from build123d import *

# Parameters (mm, degrees)
SKETCH1_R           = 79.5
BOSS_EXTRUDE1_DEPTH = 37
SKETCH2_W           = 80
SKETCH2_H           = 31
BOSS_EXTRUDE2_DEPTH = 212.65
BOSS_EXTRUDE3_DEPTH = 31
CUT_EXTRUDE1_DEPTH  = 10
SKETCH5_R           = 27.5
CUT_EXTRUDE2_DEPTH  = 181


with BuildPart() as part:
    # Sketch1 → Boss-Extrude1 (new body)
    with BuildSketch(Plane.XY):
        with BuildLine():
            ThreePointArc((-21.261874522, 100), (-28.188531545, 98.000973706), (-32.984947104, 92.618680381))
            Line((-32.984947104, 92.618680381), (-71.691097716, 11.860391562))
            ThreePointArc((-71.691097716, 11.860391562), (0, 57), (71.691097716, 11.860391562))
            Line((71.691097716, 11.860391562), (32.984947104, 92.618680381))
            ThreePointArc((32.984947104, 92.618680381), (28.188531545, 98.000973706), (21.261874522, 100))
            Line((21.261874522, 100), (-21.261874522, 100))
        make_face()
        with Locations((0, -22.5)):
            Circle(SKETCH1_R)
    extrude(amount=BOSS_EXTRUDE1_DEPTH)

    # Sketch2 → Boss-Extrude2 (add)
    with BuildSketch(Plane.XY.offset(37)):
        with Locations((0, 62.5)):
            Rectangle(SKETCH2_W, SKETCH2_H)
    extrude(amount=BOSS_EXTRUDE2_DEPTH)

    # Sketch3 → Boss-Extrude3 (add)
    with BuildSketch(Plane(origin=(0, 78, 0), x_dir=(1, 0, 0), z_dir=(0, 1, 0))):
        Polygon((5, -278.784714132), (40, -270.85), (40, -249.65), (-40, -249.65), (-40, -270.85), align=None)
    extrude(amount=-BOSS_EXTRUDE3_DEPTH)

    # Sketch4 → Cut-Extrude1 (cut)
    with BuildSketch(Plane.XY.offset(37)):
        Polygon((55, -22.5), (15, 15), (15, -7.5), (-50, -7.5), (-50, -37.5), (15, -37.5), (15, -60), align=None)
    extrude(amount=-CUT_EXTRUDE1_DEPTH, mode=Mode.SUBTRACT)

    # Sketch5 → Cut-Extrude2 (cut, through all)
    with BuildSketch(Plane(origin=(0, 78, 0), x_dir=(1, 0, 0), z_dir=(0, 1, 0))):
        with Locations((0, -206.1)):
            Circle(SKETCH5_R)
    extrude(amount=-CUT_EXTRUDE2_DEPTH, mode=Mode.SUBTRACT)


solid = part.part
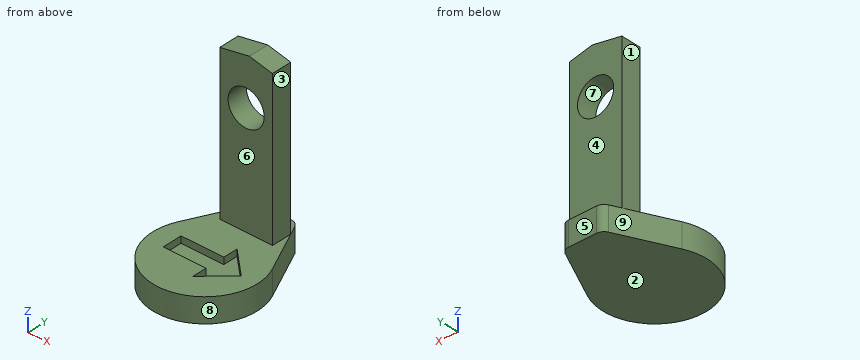
Read the model definition and answer for the solid it produces. Units are mm, in the model's axes. Face numbers are marked on the shaded views. A direction names the side the tool comes from. Round coordinates to 2 decimals unless told otherwise and drop trailing zeros. Order: outer loops, then holes, each group sorted by start corner. A loop starts at its lowest first (then second) coordinate and runs counter-clockwise, first axis right, second up.
1) Straight lines are drawn through the part: L1, parallel to X at y = 57.5, z = 206.1; L2, parallel to Y at x = -12.5, z = 155; L3, parallel to Z at x = 45, y = 19. For each, find the intervals that lie inside material, in ascending order.
2) The mould has two halves that part along X. Classify the marked faces 6, 7, 8 and 9: released by +X, released by -X, zero draft, split by the parting line, or undercut.
3) The part is cut by section C-C on z = 145. Write down the section's boundary in (x, y), plus the area to 3 significant figures.
4) For the marked faces 1, 2, 3, 4 and 5, determine the directions among +Z, -Z, +X, -X, +Y, -Y from which every point of the face is accessible in a straight line to the end or side of a thin tool.
5) Flat-ended cylindrical pins translate along their axes: pin 1 (15.5 mm diameter, centred on y = 55, z = 205, fed in from -X); pin 2 (5 mm diameter, centred on y = -47.5, z = 32.5, fed in from +X); pin 3 (5 mm diameter, centred on y = -1, z = 31, fed in from +X); pin 4 (5 mm diameter, centred on y = -25, z = 29.5, fed in from +X). Find the tip coordinate at first contact, or state that the pin passes through.
6) The part is cut by section A-A on z = 206.1. Write down the section's boundary in (x, y).
7) The part is cut by section B-B on x = 0. Write down the section's boundary in (y, z), plus the area to 3 significant figures.
8) The part is cut by section D-D on x = 60.5. Write down the section's boundary in (y, z).
Resolved:
1. L1: x = -40 to -27.5, 27.5 to 40
1. L2: y = 47 to 78
1. L3: z = 0 to 37
2. face 6: zero draft
2. face 7: undercut
2. face 8: split by the parting line
2. face 9: released by -X
3. outline: (-40, 47) - (40, 47) - (40, 78) - (-40, 78) - close
3. area: 2,480 mm2
4. face 1: +Z, -X, +Y, -Y
4. face 2: -Z, +X, -X, +Y, -Y
4. face 3: +Z, +X, +Y, -Y
4. face 4: +Z, +X, -X, +Y
4. face 5: +Z, -Z, +X, -X, +Y
5. pin 1: stops at x = -40
5. pin 2: stops at x = 76.25
5. pin 3: stops at x = 77.2
5. pin 4: stops at x = 79.5
6. outline: (-40, 47) - (-27.5, 47) - (-27.5, 78) - (-40, 78) - close; (27.5, 47) - (40, 47) - (40, 78) - (27.5, 78) - close
7. outline: (-102, 0) - (100, 0) - (100, 37) - (78, 37) - (78, 178.6) - (47, 178.6) - (47, 37) - (-7.5, 37) - (-7.5, 27) - (-37.5, 27) - (-37.5, 37) - (-102, 37) - close; (47, 233.6) - (78, 233.6) - (78, 277.9) - (47, 277.9) - close
7. area: 12,900 mm2
8. outline: (-74.08, 0) - (35.21, 0) - (35.21, 37) - (-74.08, 37) - close
